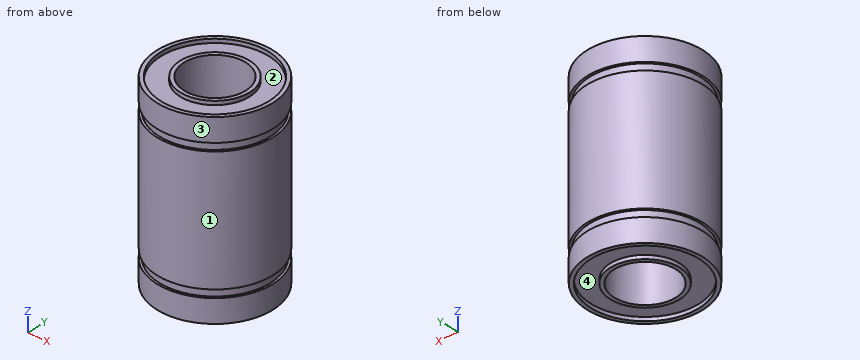
```python
from build123d import *

# Parameters (mm, degrees)
F0_R     = 7.5
F0_R_2   = 4
F1_DEPTH = 24
F2_W     = 2.5912171826
F2_H     = 1
F4_R     = 7
F4_R_2   = 4.5
F5_DEPTH = 0.5


# Not quite as in the source:
# - a pattern or mirror of a feature is missing from the dataset's text; its kind, count and spacing are read off the source's solid


with BuildPart() as f1:
    # F0 (on Top) → F1 (new body)
    with BuildSketch(Plane.XY):
        Circle(F0_R)
        Circle(F0_R_2, mode=Mode.SUBTRACT)
    extrude(amount=F1_DEPTH)

    # F2 (on Right) → F3 (revolve, cut)
    with BuildSketch(Plane.YZ):
        with Locations((8.5017232858, 20.5)):
            Rectangle(F2_W, F2_H)
        with Locations((8.5017232858, 3.5)):
            Rectangle(F2_W, F2_H)
    revolve(axis=Axis((0, 0, 24), (0, 0, 1)), mode=Mode.SUBTRACT)

    # F4 (on face) → F5 (cut)
    with BuildSketch(Plane.XY.offset(24)):
        Circle(F4_R)
        Circle(F4_R_2, mode=Mode.SUBTRACT)
    f5 = extrude(amount=-F5_DEPTH, mode=Mode.SUBTRACT)

    # F5_copies: F5 across plane
    add(f5.mirror(Plane(origin=(0, 0, 12), x_dir=(-1, 0, 0), z_dir=(0, 0, -1))), mode=Mode.SUBTRACT)


solid = f1.part
```
Design review of the part built by this model. Coordinates are the model's own, in mm. Face numbers are marked on the shaded views. A direction names the side the tool comes from. Coordinates: 2 decimals unless noted, no trailing zeros. Order: outer loops, then holes, each group sorted by start corner. A loop starts at its lowest first (then second) coordinate and runs counter-clockwise, first axis right, second up.
1) Clearance check with flat-ended pins moving along their axes: pin 1 (4.5 mm diameter, centred on x = 1, y = 1, fed in from -Z); pin 2 (8 mm diameter, centred on x = -3.5, y = -3.5, fed in from +Z). State where each tip first meets the part, or that it passes through.
2) Mouldability with a two-part tool opening along X and no side actions: class the marked faces 1 and 2 as +X half, -X half, draft (parallel to the pull), parting line (faces both ways), or undercut.
3) For the marked faces 3 and 4, list the 3-axis set-ups (+Z, -Z, +X, -X, +Y, -Y) from which the entire face can be reached by the end or side of a thin tool; tool diameter is ignored.
4) Wall thickness on line 1 along Y through (x, z) = (0, 0.35); line 2 along Y through (x, z) = (0, 17.25); line 3 along X through (y, z) = (3.5, 17): over which ranges is each line inside the solid? List them lowest first.
5) Take a section at A-A, the plane z = 22.25. Give the boundary of the cut face in (x, y).
Returned:
1. pin 1: passes through
1. pin 2: stops at z = 24
2. face 1: parting line
2. face 2: undercut
3. face 3: +Z, -Z
3. face 4: -Z
4. line 1: y = -7.5 to -7, -4.5 to -4, 4 to 4.5, 7 to 7.5
4. line 2: y = -7.5 to -4, 4 to 7.5
4. line 3: x = -6.63 to -1.94, 1.94 to 6.63
5. outline: circle Ø15 at (0, 0); hole circle Ø8 at (0, 0)
